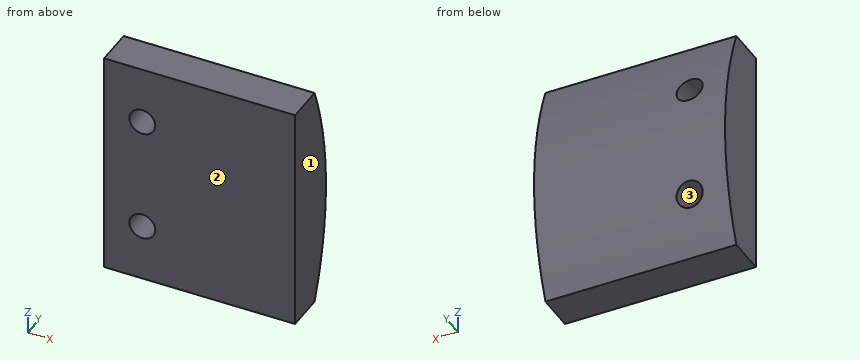
Autodesk Inventor part; units mm, degrees
ref_plane "YZ Plane" through (0, 0, 0) normal (1, 0, 0) x (0, 1, 0)
ref_plane "XZ Plane" through (0, 0, 0) normal (0, 1, 0) x (-1, 0, 0)
ref_plane "XY Plane" through (0, 0, 0) normal (0, 0, 1) x (1, 0, 0)
sketch "Sketch1" plane through (0, 0, 0) normal (1, 0, 0) x (0, 1, 0)
  line L0 (0, 0) -> (-3.175, 0)
  line L1 (-3.175, 0) -> (-3.175, -19.05)
  line L2 (-3.175, -19.05) -> (0, -19.05)
  arc A0 (0, -19.05) -> (0, 0) centre (-23.5464, -9.525) ccw
  dimension "d4" = 3.175
  dimension "d6" = 25.4
  dimension "d7" = 19.05
  dimension "d23" = 3.175
extrude "Extrusion1" add sketch "Sketch1" along normal blind 15.875
sketch "Sketch2" plane through (0, -3.175, -19.05) normal (0, -1, 0) x (1, 0, 0)
  line L0 (0, 19.05) -> (0, 0)
  line L1 (0, 0) -> (15.875, 0)
  line L2 (15.875, 19.05) -> (15.875, 0)
  line L3 (0, 19.05) -> (15.875, 19.05)
  point P0 (3.175, 14.2875)
  point P1 (3.175, 4.7625)
  dimension "d10" = 15.875
  dimension "d13" = 9.525
  dimension "d14" = 19.05
  dimension "d15" = 4.7625
  dimension "d24" = 3.175
  dimension "d25" = 3.175
hole "Hole1" at (3.175, -3.175, -4.7625) at (3.175, -3.175, -14.2875) direction (0, 1, 0) diameter 2.159 depth 6.35 tip angle 118
equation "\"d23\" = d4"
properties part number "TensionerPusher3" material "ABS Plastic"
The listing builds one solid part. Answer for the finished solid, in the listing's coordinates (mm). Face numbers are marked on the shaded views. Give positions to 0.01 mm unless a question says otherwise; leave off trailing zeros. Write each loop counter-clockwise with the first axis right and the second up, starting at its lowest first coordinate (ties: lowest second). Pieces come first, ordered by that corner, then holes. Notation, with made-up numbers: (8, 55.25) -> (55, 55.25) arc R34 cw to (55, 87.25) -> close; hole circle Ø7 at (80.5, -12). An arc over 180 degrees is marked (long way). Write item = value, one per line. Start each with the question number.
1) The part is cut by section C-C, the plane y = 0.45. Determine the outline of the cut face in (x, z) (1 decimal), and give its area (3 significant figures).
2) The part is cut by section A-A, the plane x = 3.75. Determine the outline of the cut face in (y, z) (3 decimals).
3) The part is cut by section B-B, the plane z = -5.5. Determine the outline of the cut face in (x, y) (3 decimals).
4) Determine the mould class of the marked faces 1, 2 and 3 for opening direction X: +X half, -X half, draft (parallel to the pull), parting line (faces both ways), or undercut.
5) Each of these flat-tipped pins is pushed along its axis until it touches: pin 1 (6 mm diameter, centred on x = 9.5, z = -2.5, fed in from +Y); pin 2 (3 mm diameter, centred on x = 3.18, z = -4.76, fed in from +Y); pin 3 (1.7 mm diameter, centred on x = 3.18, z = -14.29, fed in from -Y). Where does it stop, or does it pass through?
6) Straight lines are drawn through the part: line 1 along Z through (x, y) = (2.75, -1.3); line 2 along Z through (x, y) = (3, -1.8); line 3 along X through (y, z) = (0.05, -4) (3 decimals). For each, find the intervals that lie inside material, in ascending order.
7) The part is cut by section D-D, the plane x = 11.75. Determine the outline of the cut face in (y, z) (3 decimals).
Solutions:
q1.outline = (0, -17.9) -> (15.9, -17.9) -> (15.9, -1.2) -> (0, -1.2) -> close; hole circle Ø2.2 at (3.2, -14.3); hole circle Ø2.2 at (3.2, -4.8)
q1.area = 257 mm²
q2.outline = (-3.175, -19.05) -> (0, -19.05) arc R25.4 ccw to (1.211, -15.201) -> (-3.175, -15.201) -> close; (-3.175, -13.374) -> (1.56, -13.374) arc R25.4 ccw to (1.56, -5.676) -> (-3.175, -5.676) -> close; (-3.175, -3.849) -> (1.211, -3.849) arc R25.4 ccw to (0, 0) -> (-3.175, 0) -> close
q3.outline = (0, -3.175) -> (2.387, -3.175) -> (2.387, 1.533) -> (0, 1.533) -> close; (3.963, -3.175) -> (15.875, -3.175) -> (15.875, 1.533) -> (3.963, 1.533) -> close
q4.face_1 = +X half
q4.face_2 = draft
q4.face_3 = undercut
q5.pin_1 = 1.53
q5.pin_2 = 1.64
q5.pin_3 = through
q6.line_1 = -19.05 to -15.28, -13.3 to -5.75, -3.77 to 0
q6.line_2 = -19.05 to -15.35, -13.22 to -5.83, -3.7 to 0
q6.line_3 = 0 to 2.411, 3.939 to 15.875
q7.outline = (-3.175, -19.05) -> (0, -19.05) arc R25.4 ccw to (0, 0) -> (-3.175, 0) -> close
